Work out the finished part from the listing and answer in its coordinate system (mm). Face numbers are marked on the shaded views. Give positions to 0.01 mm unless a question says otherwise; leave off trailing zeros. Order: outer loops, then holes, each group sorted by start corner. A loop starts at its lowest first (then second) coordinate and runs counter-clockwise, first axis right, second up. Notation, with made-up numbers: (-15, 71.25) - (24, 71.25) arc R17 cw to (24, 81.25) - close; hole circle Ø8 at (45.5, 42.5). An arc over 180 degrees is marked (long way). Put each result on its own line as item: value.
```python
from build123d import *

# Parameters (mm, degrees)
F0_R     = 11.075
F1_DEPTH = 7.1
F2_R     = 1.8


with BuildPart() as f1:
    # F0 (on Top) → F1 (new body)
    with BuildSketch(Plane.XY):
        with BuildLine():
            ThreePointArc((10.883850477, 28.6876300688), (9.4184768424, 23.182114097), (5.4101337969, 19.1335079129))
            Line((5.4101337969, 19.1335079129), (6.5345129791, 17.2156516926))
            Line((6.5345129791, 17.2156516926), (13.1067064335, 21.0101093527))
            Line((13.1067064335, 21.0101093527), (13.1067064335, 36.365150785))
            Line((13.1067064335, 36.365150785), (-0.191149523, 44.0426715011))
            Line((-0.191149523, 44.0426715011), (-13.4890054796, 36.365150785))
            Line((-13.4890054796, 36.365150785), (-13.4890054796, 21.0101093527))
            Line((-13.4890054796, 21.0101093527), (-6.7633429774, 17.1270462966))
            Line((-6.7633429774, 17.1270462966), (-5.664620361, 19.059715342))
            ThreePointArc((-5.664620361, 19.059715342), (-5.7605720905, 38.2603599441), (10.883850477, 28.6876300688))
        make_face()
        with BuildLine():
            Line((6.5345129791, 17.2156516926), (5.4101337969, 19.1335079129))
            ThreePointArc((5.4101337969, 19.1335079129), (-0.1173569522, 17.612875911), (-5.664620361, 19.059715342))
            Line((-5.664620361, 19.059715342), (-6.7633429774, 17.1270462966))
            Line((-6.7633429774, 17.1270462966), (-0.191149523, 13.3325886365))
            Line((-0.191149523, 13.3325886365), (6.5345129791, 17.2156516926))
        make_face()
        Polygon((18.2140135788, -2.7060999984), (6.5345129791, 17.2156516926), (-0.191149523, 13.3325886365), (-6.7633429774, 17.1270462966), (-18.1763357298, -2.9485737718), (-11.4438602402, -6.8435092462), (-11.4505581332, -14.420748465), (11.6417076562, -14.2668816039), (11.5340385205, -6.6904044278), align=None)
        Circle(F0_R, mode=Mode.SUBTRACT)
        with BuildLine():
            Line((24.7216007166, 1.1753827964), (18.2140135788, -2.7060999984))
            Line((18.2140135788, -2.7060999984), (19.3385078556, -4.6241525356))
            ThreePointArc((19.3385078556, -4.6241525356), (30.4453071473, -4.5686483261), (36.0147911755, -14.1782746915))
            ThreePointArc((36.0147911755, -14.1782746915), (24.9766876657, -25.2532132308), (13.8650370177, -14.2520672624))
            Line((13.8650370177, -14.2520672624), (11.6417076562, -14.2668816039))
            Line((11.6417076562, -14.2668816039), (11.7522289794, -22.0440619158))
            Line((11.7522289794, -22.0440619158), (25.1579816344, -29.5319321795))
            Line((25.1579816344, -29.5319321795), (38.3455438305, -21.6661449552))
            Line((38.3455438305, -21.6661449552), (38.1273533716, -6.3124874673))
            Line((38.1273533716, -6.3124874673), (24.7216007166, 1.1753827964))
        make_face()
        with BuildLine():
            Line((19.3385078556, -4.6241525356), (18.2140135788, -2.7060999984))
            Line((18.2140135788, -2.7060999984), (11.5340385205, -6.6904044278))
            Line((11.5340385205, -6.6904044278), (11.6417076562, -14.2668816039))
            Line((11.6417076562, -14.2668816039), (13.8650370177, -14.2520672624))
            ThreePointArc((13.8650370177, -14.2520672624), (15.3118764487, -8.7048038536), (19.3385078556, -4.6241525356))
        make_face()
        with BuildLine():
            Line((-11.4438602402, -6.8435092462), (-18.1763357298, -2.9485737718))
            Line((-18.1763357298, -2.9485737718), (-19.2751708145, -4.8814406505))
            ThreePointArc((-19.2751708145, -4.8814406505), (-15.1945194965, -8.9080720574), (-13.6738874946, -14.4355628064))
            Line((-13.6738874946, -14.4355628064), (-11.4505581332, -14.420748465))
            Line((-11.4505581332, -14.420748465), (-11.4438602402, -6.8435092462))
        make_face()
        with BuildLine():
            Line((-19.2751708145, -4.8814406505), (-18.1763357298, -2.9485737718))
            Line((-18.1763357298, -2.9485737718), (-24.7350684373, 0.8458463831))
            Line((-24.7350684373, 0.8458463831), (-38.0398498496, -6.819999748))
            Line((-38.0398498496, -6.819999748), (-38.0534230647, -22.1752015083))
            Line((-38.0534230647, -22.1752015083), (-24.7622148676, -29.8645571376))
            Line((-24.7622148676, -29.8645571376), (-11.4574334553, -22.1987110066))
            Line((-11.4574334553, -22.1987110066), (-11.4505581332, -14.420748465))
            Line((-11.4505581332, -14.420748465), (-13.6738874946, -14.4355628064))
            ThreePointArc((-13.6738874946, -14.4355628064), (-13.6737031132, -14.4724588871), (-13.6736416525, -14.5093553773))
            ThreePointArc((-13.6736416525, -14.5093553773), (-34.3213715277, -20.0787779447), (-19.2751708145, -4.8814406505))
        make_face()
    extrude(amount=F1_DEPTH)

    # F2
    f2_edges = [f1.edges().sort_by_distance(p)[0] for p in [
        (-18.109824, -26.031634, 7.1),
        (0.095575, -14.343815, 7.1),
        (18.455105, -25.787997, 7.1),
        (31.751763, -25.599039, 7.1),
        (38.236449, -13.989316, 7.1),
        (31.424477, -2.568552, 7.1),
        (21.467807, -0.765359, 7.1),
        (12.374263, 7.254776, 7.1),
        (-31.407819, -26.019879, 7.1),
        (-38.046636, -14.497601, 7.1),
        (-31.387459, -2.987077, 7.1),
        (-21.455702, -1.051364, 7.1),
        (-12.469839, 7.089236, 7.1),
        (-10.126174, 19.068578, 7.1),
        (-13.489005, 28.68763, 7.1),
        (-6.840078, 40.203911, 7.1),
        (6.457778, 40.203911, 7.1),
        (13.106706, 28.68763, 7.1),
        (9.82061, 19.112881, 7.1),
        (31.424477, -2.568552, 0),
        (21.467807, -0.765359, 0),
        (12.374263, 7.254776, 0),
        (9.82061, 19.112881, 0),
        (13.106706, 28.68763, 0),
        (6.457778, 40.203911, 0),
        (-6.840078, 40.203911, 0),
        (-13.489005, 28.68763, 0),
        (-10.126174, 19.068578, 0),
        (-12.469839, 7.089236, 0),
        (-21.455702, -1.051364, 0),
        (-31.387459, -2.987077, 0),
        (-38.046636, -14.497601, 0),
        (-31.407819, -26.019879, 0),
        (-18.109824, -26.031634, 0),
        (-11.453996, -18.30973, 0),
        (0.095575, -14.343815, 0),
        (11.696968, -18.155472, 0),
        (18.455105, -25.787997, 0),
        (31.751763, -25.599039, 0),
        (38.236449, -13.989316, 0),
        (-11.453996, -18.30973, 7.1),
        (11.696968, -18.155472, 7.1),
    ]]
    fillet(f2_edges, radius=F2_R)


solid = f1.part
```
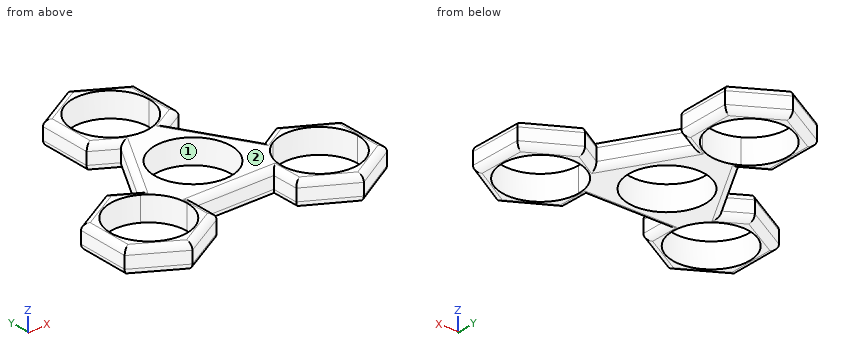
(1) Determine the mould class of the marked faces 1 and 2 for opening direction Y: pulls with the +Y half, pulls with the -Y half, needs draft (parallel to the pull), parting line crosses it, or undercut.
Geometry check:
face 1: undercut
face 2: needs draft
(2) Given pin 1 (4 mm diameter, centred on y = -20, z = 1.5, fed in from -X); pin 2 (1.8 mm diameter, centred on y = 30, z = 3.5, fed in from +X); pin 3 (1.5 mm diameter, centred on x = 20.5, z = 3.5, fed in from -Y); pin 4 (4 mm diameter, centred on x = 0.5, z = 2, fed in from -Y), each flat-ended and moving along its own axis, determine where each tip first touches the part or whether it passes through.
Geometry check:
pin 1: stops at x = -38.05
pin 2: stops at x = 13.11
pin 3: stops at y = -27.35
pin 4: stops at y = -14.35
(3) Straight lines are drawn through the part: line 1 (Y direction, x = 3, z = 0.75); line 2 (X direction, y = -20.5, z = 5.75); line 3 (Y direction, x = -4, z = 0.75). For each, find the intervals that lie inside material, in ascending order.
Geometry check:
line 1: y = -13.99 to -10.66, 10.66 to 18.08, 39.29 to 41.81
line 2: x = -37.99 to -34.06, -15.43 to -11.51, 11.79 to 15.85, 34.03 to 38.27
line 3: y = -14.03 to -10.33, 10.33 to 18.29, 39.09 to 41.45
(4) Section A-A, the plane z = 2.75 is taken. Count the separate pieces of the cut face and the enclosed holes in it, then the cut area to 3 significant figures.
Geometry check:
separate pieces: 1
enclosed holes: 4
area: 1,060 mm²
(5) Section B-B, the plane y = 25.5 is taken. Write down the section's boundary in (x, z), then the cut area to 3 significant figures.
Geometry check:
outline: (-13.49, 1.8) arc R1.8 ccw to (-11.69, 0) - (-10.8, 0) - (-10.8, 7.1) - (-11.69, 7.1) arc R1.8 ccw to (-13.49, 5.3) - close; (10.42, 0) - (11.31, 0) arc R1.8 ccw to (13.11, 1.8) - (13.11, 5.3) arc R1.8 ccw to (11.31, 7.1) - (10.42, 7.1) - close
area: 35.4 mm²
